from build123d import *

# Parameters (mm, degrees)
SALIENTE_EXTRUIR1_DEPTH = 3
REDONDEO1_R             = 3
REDONDEO2_R             = 1.5
CROQUIS3_R              = 1.475
CORTAR_EXTRUIR1_DEPTH   = 15.812114009
CROQUIS4_R              = 0.75
CORTAR_EXTRUIR2_DEPTH   = 15.565263254


with BuildPart() as part:
    # Croquis1 → Saliente-Extruir1 (new, symmetric)
    with BuildSketch(Plane.XY):
        Polygon((0, 0), (-7.498427125, 0), (-13.274377336, 5.775950212), (-11.860163774, 7.190163774), (-6.67, 2), (0, 2), align=None)
    extrude(amount=SALIENTE_EXTRUIR1_DEPTH, both=True)

    # Redondeo1
    redondeo1_edges = [part.edges().sort_by_distance(p)[0] for p in [
        (-12.567270555, 6.483056993, -3),
        (-12.567270555, 6.483056993, 3),
    ]]
    fillet(redondeo1_edges, radius=REDONDEO1_R - 0.0001)  # a hair under: the kernel refuses the full size

    # Redondeo2
    redondeo2_edges = [part.edges().sort_by_distance(p)[0] for p in [
        (0, 1, 3),
        (0, 1, -3),
    ]]
    fillet(redondeo2_edges, radius=REDONDEO2_R)

    # Croquis3 → Cortar-Extruir1 (cut, through all)
    with BuildSketch(Plane(origin=(-2.335, -2.335, 0), x_dir=(0, 0, -1), z_dir=(0.7071067811865485, 0.7071067811865466, 0))):
        with Locations(Location((0, 10.470615793, 0), (0, 0, 90))):
            Circle(CROQUIS3_R)
    extrude(amount=-CORTAR_EXTRUIR1_DEPTH, mode=Mode.SUBTRACT)

    # Croquis4 → Cortar-Extruir2 (cut, through all)
    with BuildSketch(Plane(origin=(0, 2, 0), x_dir=(1, 0, 0), z_dir=(0, 1, 0))):
        with Locations(Location((-5, 0, 0), (0, 0, 180))):
            Circle(CROQUIS4_R)
        with Locations(Location((-2, 0, 0), (0, 0, 180))):
            Circle(CROQUIS4_R)
    extrude(amount=-CORTAR_EXTRUIR2_DEPTH, mode=Mode.SUBTRACT)


solid = part.part
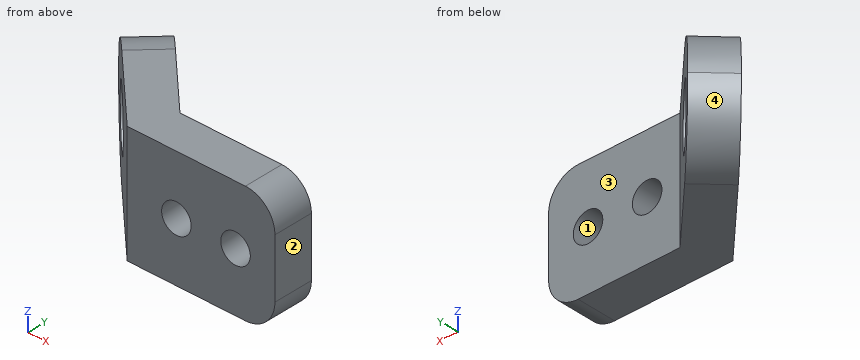
Check sheet for the modelled part. Datum: model origin and axes. Units: mm. Face numbers are marked on the shaded views. Round coordinates to 2 decimals unless told otherwise and drop trailing zeros. Loops run counter-clockwise (first coordinate to the right, second up) from the corner with the lowest first, then second, coordinate; pieces in that order, holes last. Notation, with made-up numbers: (-15, 20) -> (31, 20) arc R11 cw to (31, 31) -> close; hole circle Ø2 at (63, -28). An arc over 180 degrees is marked (long way). Put each result on its own line as item: value. Start each with the question number.
1. Section check D-D (z = 1.25). Enter the section's corners in (x, y).
2. Section check A-A (x = -5). Enter the section's corners in (y, z).
3. Section check C-C (z = 2). Enter the section's corners in (x, y).
4. Draft check along X on the marked faces 1, 2, 3 and 4. Enter one of: +X half, -X half, draft (parallel to the pull), parting line (faces both ways), or undercut.
5. Scan lines: probe 1 along Z at (x, y) = (-2, 1); probe 2 along Y at (x, z) = (-5.5, -2.25); probe 3 along X at (y, z) = (6.5, -0.5). Record each from-to range of solid material in increasing order.
6. Section check B-B (z = -1). Enter the section's corners in (x, y).
7. Gauge pin test, flat ends, axial feed: pin 1 (2 mm diameter, centred on x = -6, y = 3.5, fed in from +Z); pin 2 (2 mm diameter, centred on x = -11, z = 0, fed in from +Y); pin 3 (1.5 mm diameter, centred on y = 1, z = -1.5, fed in from -X); pin 4 (2 mm diameter, centred on x = -5, z = 0, fed in from +Y). Record the tip position at first contact, or that the pin passes through.
Findings:
1. outline: (-13.08, 5.58) -> (-11.71, 4.21) -> (-10.29, 5.62) -> (-11.67, 7) -> close; (-10.6, 3.1) -> (-7.5, 0) -> (0, 0) -> (0, 2) -> (-6.67, 2) -> (-9.19, 4.52) -> close
2. outline: (0, -3) -> (2, -3) -> (2, -0.75) -> (0, -0.75) -> close; (0, 0.75) -> (2, 0.75) -> (2, 3) -> (0, 3) -> close
3. outline: (-12.73, 5.24) -> (-7.5, 0) -> (-0.09, 0) -> (-0.09, 2) -> (-6.67, 2) -> (-11.32, 6.65) -> close
4. face 1: undercut
4. face 2: +X half
4. face 3: draft
4. face 4: -X half
5. probe 1: z = -3 to -0.75, 0.75 to 3
5. probe 2: y = 0 to 2
5. probe 3: x = -12.49 to -11.17
6. outline: (-13.15, 5.65) -> (-11.92, 4.42) -> (-10.51, 5.84) -> (-11.74, 7.07) -> close; (-10.39, 2.89) -> (-7.5, 0) -> (0, 0) -> (0, 2) -> (-6.67, 2) -> (-8.97, 4.3) -> close
7. pin 1: passes through
7. pin 2: stops at y = 7.19
7. pin 3: stops at x = -9.25
7. pin 4: stops at y = 2
